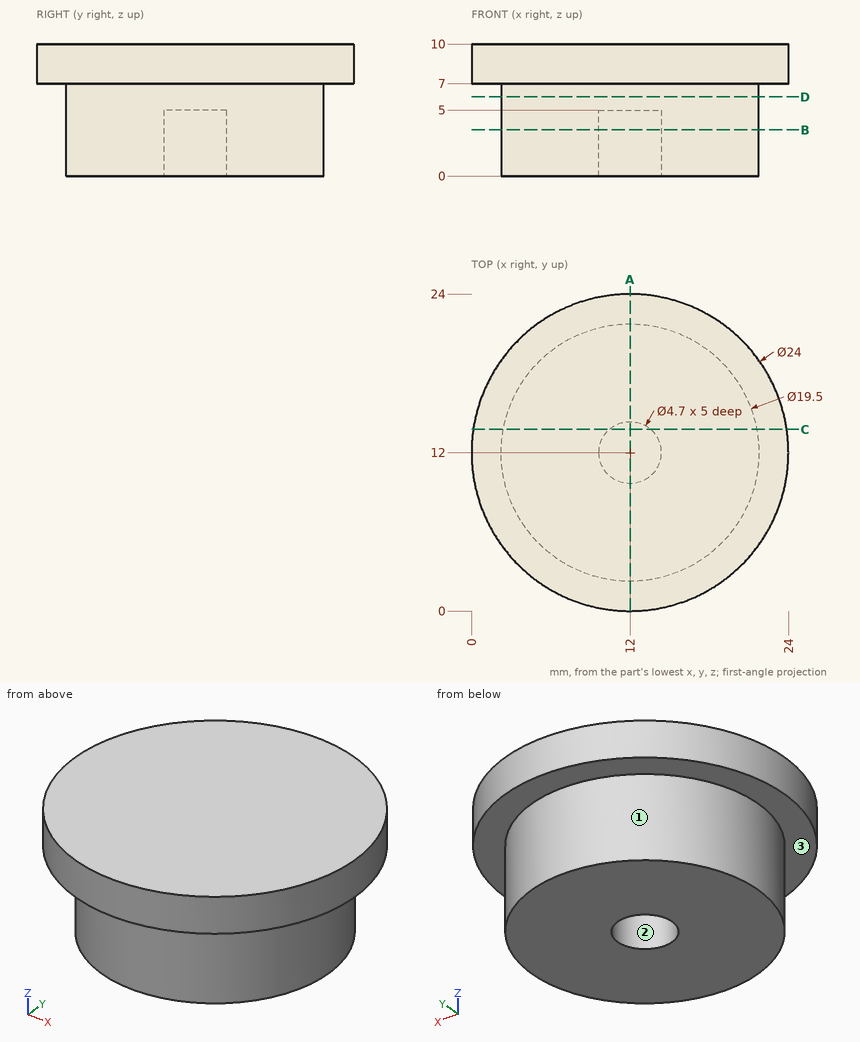
Could you check a few things on this drawing? It's one solid part, dimensions in mm from its lowest x, y, z. Round coordinates to 2 decimals unless told otherwise and drop trailing zeros. Write each loop counter-clockwise with the first axis right and the second up, starting at its lowest first coordinate (ties: lowest second). Pieces come first, ordered by that corner, then holes. Notation, with made-up numbers: (62.5, 42) -> (114.5, 42) arc R19 cw to (114.5, 64) -> close; hole circle Ø9 at (59, 28.25). An arc over 180 degrees is marked (long way). Use a Markdown table: item, result.
1. For pin 1 Ø6 at (y, z) = (5, 4.5) entering from +X; pin 2 Ø4 at (x, y) = (13, 13) entering from -Z; pin 3 Ø4 at (y, z) = (10, 2) entering from +X, each with a flat end and sliding along its axis, tell me the tip position at first contact or that it passes through.
Answer key:
| item | result |
|---|---|
| pin 1 | stops at x = 22.75 |
| pin 2 | stops at z = 0 |
| pin 3 | stops at x = 21.75 |
2. If we section it at B-B (z = 3.5): List the corners of the cut face in (x, y) for me, then the cut area to 3 significant figures.
Answer key:
| item | result |
|---|---|
| outline | circle Ø19.5 at (12, 12); hole circle Ø4.7 at (12, 12) |
| area | 281 mm^2 |
3. Please list where these lines run through material, in increasing order: probe 1 along Z at (x, y) = (1.25, 7.75); probe 2 along Y at (x, z) = (12, 2.6); probe 3 along Y at (x, z) = (10.5, 4).
Answer key:
| item | result |
|---|---|
| probe 1 | z = 7 to 10 |
| probe 2 | y = 2.25 to 9.65, 14.35 to 21.75 |
| probe 3 | y = 2.37 to 10.19, 13.81 to 21.63 |
4. If we section it at A-A (x = 12): List the corners of the cut face in (y, z) for me.
Answer key:
| item | result |
|---|---|
| outline | (0, 7) -> (2.25, 7) -> (2.25, 0) -> (9.65, 0) -> (9.65, 5) -> (14.35, 5) -> (14.35, 0) -> (21.75, 0) -> (21.75, 7) -> (24, 7) -> (24, 10) -> (0, 10) -> close |
5. If we section it at D-D (z = 6): List the corners of the cut face in (x, y) for me.
Answer key:
| item | result |
|---|---|
| outline | circle Ø19.5 at (12, 12) |
6. If we section it at C-C (y = 13.75): List the corners of the cut face in (x, z) for me, then the cut area to 3 significant figures.
Answer key:
| item | result |
|---|---|
| outline | (0.13, 7) -> (2.41, 7) -> (2.41, 0) -> (10.43, 0) -> (10.43, 5) -> (13.57, 5) -> (13.57, 0) -> (21.59, 0) -> (21.59, 7) -> (23.87, 7) -> (23.87, 10) -> (0.13, 10) -> close |
| area | 190 mm^2 |
7. We'd pull the mould along Y, two halves only. Please class the marked faces 1, 2 and 3: +Y half, -Y half, draft (parallel to the pull), parting line (faces both ways), or undercut.
Answer key:
| item | result |
|---|---|
| face 1 | parting line |
| face 2 | undercut |
| face 3 | draft |
